Here's how the part is built. I have some questions about the finished solid (model axes, mm). A direction names the side the tool comes from. Give positions to 0.01 mm unless a question says otherwise; leave off trailing zeros. Write each loop counter-clockwise with the first axis right and the second up, starting at its lowest first coordinate (ties: lowest second). Pieces come first, ordered by that corner, then holes. Notation, with made-up numbers: (-32, 77.25) - (26, 77.25) arc R34 cw to (26, 115.25) - close; hole circle Ø4 at (63.5, -2.75). An arc over 180 degrees is marked (long way). Use a Markdown table: item, result.
```python
from build123d import *

# Parameters (mm, degrees)
SKETCH1_R               = 20
BOSS_EXTRUDE1_DEPTH     = 40
SKETCH2_W               = 10
SKETCH2_H               = 20
CUT_EXTRUDE1_DEPTH      = 40
CUT_EXTRUDE1_DEPTH_BACK = 40
SKETCH3_W               = 20
SKETCH3_H               = 10
CUT_EXTRUDE2_DEPTH      = 40
CUT_EXTRUDE2_DEPTH_BACK = 40


with BuildPart() as part:
    # Sketch1 → Boss-Extrude1 (new body)
    with BuildSketch(Plane.XY):
        Circle(SKETCH1_R)
    extrude(amount=BOSS_EXTRUDE1_DEPTH)

    # Sketch2 → Cut-Extrude1 (cut, two sides)
    with BuildSketch(Plane(origin=(0, 0, 0), x_dir=(1, 0, 0), z_dir=(0, 1, 0))) as cut_extrude1_sk:
        with Locations((-15, -20)):
            Rectangle(SKETCH2_W, SKETCH2_H)
    extrude(amount=CUT_EXTRUDE1_DEPTH, mode=Mode.SUBTRACT)
    extrude(cut_extrude1_sk.sketch, amount=-CUT_EXTRUDE1_DEPTH_BACK, mode=Mode.SUBTRACT)

    # Sketch3 → Cut-Extrude2 (cut, two sides)
    with BuildSketch(Plane(origin=(0, 0, 0), x_dir=(0, 0, -1), z_dir=(1, 0, 0))) as cut_extrude2_sk:
        with Locations((-20, 15)):
            Rectangle(SKETCH3_W, SKETCH3_H)
        with Locations((-20, -15)):
            Rectangle(SKETCH3_W, SKETCH3_H)
    extrude(amount=CUT_EXTRUDE2_DEPTH, mode=Mode.SUBTRACT)
    extrude(cut_extrude2_sk.sketch, amount=-CUT_EXTRUDE2_DEPTH_BACK, mode=Mode.SUBTRACT)


solid = part.part
```
Item 1: If we section it at D-D, the plane y = 13.5: Write out the boundary of the cut face in (x, z), plus the area to 3 significant figures.
Values:
| item | result |
|---|---|
| outline | (-14.76, 0) - (14.76, 0) - (14.76, 10) - (-14.76, 10) - close; (-14.76, 30) - (14.76, 30) - (14.76, 40) - (-14.76, 40) - close |
| area | 590 mm2 |
Item 2: For faces 4 (the flat face through (-14, 0, 30)), 5 (the flat face through (3, 10, 20)), 6 (the flat face through (3, -10, 20)), which set-ups out of +Z, -Z, +X, -X, +Y, -Y let a thin tool reach every point of the face, with its end or its side?
Values:
| item | result |
|---|---|
| face 4 | -X |
| face 5 | +X, -X, +Y |
| face 6 | +X, -X, -Y |
Item 3: I need wall thicknesses on line 1 along Z through (x, y) = (-13, -8.5); line 2 along Y through (x, z) = (4, 24); line 3 along X through (y, z) = (11, 33). Which ranges of each line are inside material? Lowest first, please. Write a range as [from, to].
Values:
| item | result |
|---|---|
| line 1 | z = [0, 10], [30, 40] |
| line 2 | y = [-10, 10] |
| line 3 | x = [-16.7, 16.7] |
Item 4: If we section it at A-A, the plane y = 0: Write out the boundary of the cut face in (x, z), plus the area to 3 significant figures.
Values:
| item | result |
|---|---|
| outline | (-20, 0) - (20, 0) - (20, 40) - (-20, 40) - (-20, 30) - (-10, 30) - (-10, 10) - (-20, 10) - close |
| area | 1,400 mm2 |
Item 5: If we section it at B-B, the plane x = -11.5: Write out the boundary of the cut face in (y, z), plus the area to 3 significant figures.
Values:
| item | result |
|---|---|
| outline | (-16.36, 0) - (16.36, 0) - (16.36, 10) - (-16.36, 10) - close; (-16.36, 30) - (16.36, 30) - (16.36, 40) - (-16.36, 40) - close |
| area | 655 mm2 |
Item 6: Thinking about a two-plate mould opening in Z: for faces 1 (the flat face through (-14, 0, 10)), 2 (the flat face through (0, 0, 40)), 3 (the flat face through (0, 0, 0)), which applies, +Z half, -Z half, draft (parallel to the pull), parting line (faces both ways), or undercut?
Values:
| item | result |
|---|---|
| face 1 | undercut |
| face 2 | +Z half |
| face 3 | -Z half |
Item 7: If we section it at C-C, the plane x = 0: Write out the boundary of the cut face in (y, z), plus the area to 3 significant figures.
Values:
| item | result |
|---|---|
| outline | (-20, 0) - (20, 0) - (20, 10) - (10, 10) - (10, 30) - (20, 30) - (20, 40) - (-20, 40) - (-20, 30) - (-10, 30) - (-10, 10) - (-20, 10) - close |
| area | 1,200 mm2 |
Item 8: Will these pins go through, and if not, where does the flat tip stop? pin 1 Ø1 at (y, z) = (-10, 17.5) entering from -X; pin 2 Ø12 at (x, y) = (4, -4) entering from -Z; pin 3 Ø10 at (x, z) = (4.5, 16.5) entering from +Y; pin 4 Ø12 at (x, z) = (-7.5, 7) entering from -Y.
Values:
| item | result |
|---|---|
| pin 1 | stops at x = -10 |
| pin 2 | stops at z = 0 |
| pin 3 | stops at y = 10 |
| pin 4 | stops at y = -19.94 |
